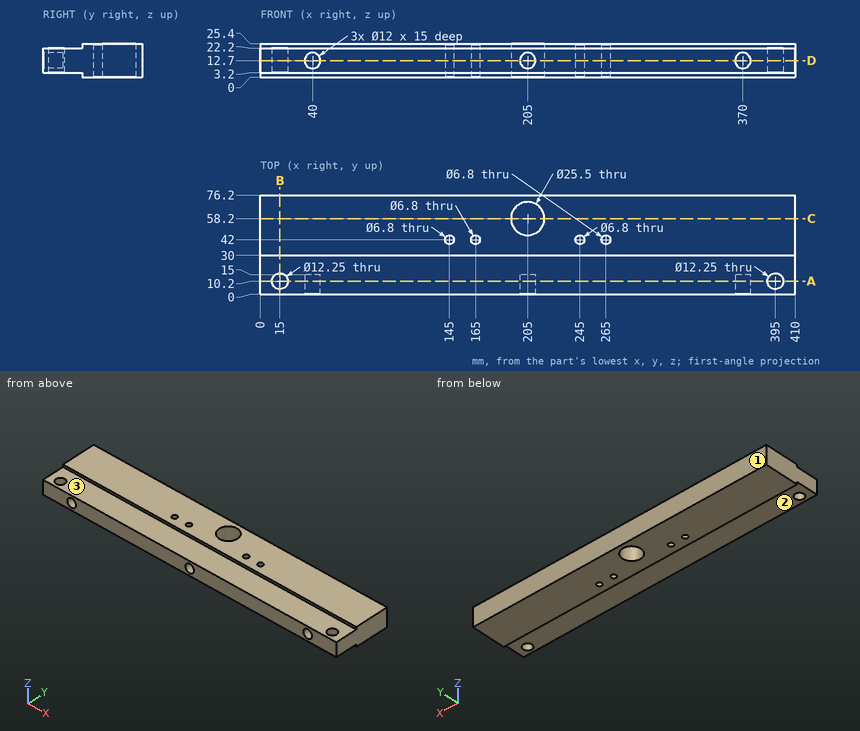
For this review, use the dimensioned drawing (mm, ordinates from the lowest corner) and the shaded views. A direction names the side the tool comes from. Give positions to 0.01 mm unless a question says otherwise; leave off trailing zeros. Order: outer loops, then holes, each group sorted by start corner. A loop starts at its lowest first (then second) coordinate and runs counter-clockwise, first axis right, second up. Notation, with made-up numbers: (16, 88.5) - (74, 88.5) arc R23 ccw to (74, 120.5) - close; hole circle Ø11 at (24.5, 82). An arc over 180 degrees is marked (long way). Use CSV: the item, a comma, the result in double quotes. Start each with the question number.
Q1. We need section C-C, the plane y = 58.2. Write out the cut boundary in (x, z), and give its area (3 significant figures).
Q2. To check wall thickness, follow line 1 along Y through (x, z) = (205, 9.25); line 2 along Z through (x, y) = (205, 7.5); line 3 along Y through (x, z) = (265, 9.5). State the ranges of each line that lie inside material, in increasing order. Write a range as [from, to].
Q3. We need section D-D, the plane z = 12.7. Write out the cut boundary in (x, y) (3 decimals).
Q4. We need section B-B, the plane x = 15. Write out the cut boundary in (y, z) (3 decimals), and give its area (3 significant figures).
Q5. We need section A-A, the plane y = 10.2. Write out the cut boundary in (x, z) (3 decimals), and give its area (3 significant figures).
Q6. Tool access review of the marked faces 1, 2 and 3: name each direction out of +Z, -Z, +X, -X, +Y, -Y from which nothing blocks a thin tool from reaching the whole face with its end or side.
Q7. Clearance check with flat-ended pins moving along their axes: pin 1 Ø5.5 at (x, y) = (245, 42) entering from -Z; pin 2 Ø14 at (x, y) = (15, 10.2) entering from -Z; pin 3 Ø1.6 at (x, z) = (200.5, 24.5) entering from -Y. State where each tip first meets the part, or that it passes through.
Outcome:
1,outline,"(0, 0) - (192.25, 0) - (192.25, 25.4) - (0, 25.4) - close; (217.75, 0) - (410, 0) - (410, 25.4) - (217.75, 25.4) - close"
1,area,"9,770 mm^2"
2,line 1,"y = [15, 45.45], [70.95, 76.2]"
2,line 2,"z = [3.2, 6.7], [18.7, 22.2]"
2,line 3,"y = [0, 38.6], [45.4, 76.2]"
3,outline,"(0, 0) - (34, 0) - (34, 15) - (46, 15) - (46, 0) - (199, 0) - (199, 15) - (211, 15) - (211, 0) - (364, 0) - (364, 15) - (376, 15) - (376, 0) - (410, 0) - (410, 76.2) - (0, 76.2) - close; hole circle Ø12.25 at (15, 10.2); hole circle Ø6.8 at (145, 42); hole circle Ø6.8 at (165, 42); hole circle Ø25.5 at (205, 58.2); hole circle Ø6.8 at (245, 42); hole circle Ø6.8 at (265, 42); hole circle Ø12.25 at (395, 10.2)"
4,outline,"(0, 3.2) - (4.075, 3.2) - (4.075, 22.2) - (0, 22.2) - close; (16.325, 3.2) - (30, 3.2) - (30, 0) - (76.2, 0) - (76.2, 25.4) - (30, 25.4) - (30, 22.2) - (16.325, 22.2) - close"
4,area,"1,510 mm^2"
5,outline,"(0, 3.2) - (8.875, 3.2) - (8.875, 22.2) - (0, 22.2) - close; (21.125, 3.2) - (388.875, 3.2) - (388.875, 22.2) - (21.125, 22.2) - close; (401.125, 3.2) - (410, 3.2) - (410, 22.2) - (401.125, 22.2) - close; hole circle Ø12 at (40, 12.7); hole circle Ø12 at (205, 12.7); hole circle Ø12 at (370, 12.7)"
5,area,"6,990 mm^2"
6,face 1,"+Z, -Z, +X, -X, +Y"
6,face 2,"-Z, +X, -X, -Y"
6,face 3,"+Z, +X, -X, -Y"
7,pin 1,"passes through"
7,pin 2,"stops at z = 3.2"
7,pin 3,"stops at y = 30"
